```python
from build123d import *

# Parameters (mm, degrees)
CROQUIS1_R                                           = 32.7
CROQUIS1_R_2                                         = 5
SALIENTE_EXTRUIR1_DEPTH                              = 4.25
REFRENTADO_PARA_TORNILLO_CON_CABEZA_TRON_D           = 3.4
REFRENTADO_PARA_TORNILLO_CON_CABEZA_TRON_CBORE_D     = 7
REFRENTADO_PARA_TORNILLO_CON_CABEZA_TRON_CBORE_DEPTH = 2.4
CROQUIS5_R                                           = 32.7
CROQUIS5_R_2                                         = 21.5
SALIENTE_EXTRUIR2_DEPTH                              = 55
TALADRO_DE_MARGEN_PARA_M31_D                         = 3.4
TALADRO_DE_MARGEN_PARA_M31_DEPTH                     = 15
TALADRO_DE_MARGEN_PARA_M31_TIP                       = 1.021463052
TALADRO_DE_MARGEN_PARA_M32_D                         = 3.4
TALADRO_DE_MARGEN_PARA_M32_DEPTH                     = 16.5
TALADRO_DE_MARGEN_PARA_M32_TIP                       = 1.021463052
CROQUIS16_R                                          = 32.7
SALIENTE_EXTRUIR3_DEPTH                              = 7.5
SALIENTE_EXTRUIR4_START                              = -10
CROQUIS17_R                                          = 42.5
CROQUIS17_R_2                                        = 32.7
SALIENTE_EXTRUIR4_DEPTH                              = 10
REFRENTADO_PARA_TORNILLO_CON_CABEZA_2_D              = 3.4
REFRENTADO_PARA_TORNILLO_CON_CABEZA_2_CBORE_D        = 7
REFRENTADO_PARA_TORNILLO_CON_CABEZA_2_CBORE_DEPTH    = 2.4


with BuildPart() as part:
    # Croquis1 → Saliente-Extruir1 (new, symmetric)
    with BuildSketch(Plane(origin=(0, 0, 0), x_dir=(0, 0, -1), z_dir=(1, 0, 0))):
        Circle(CROQUIS1_R)
        Circle(CROQUIS1_R_2, mode=Mode.SUBTRACT)
    extrude(amount=SALIENTE_EXTRUIR1_DEPTH, both=True)

    # Refrentado para tornillo con cabeza tron (through all)
    with Locations(Plane(origin=(4.25, 0, 0), x_dir=(0, 0, -1), z_dir=(1, 0, 0))):
        with Locations((8.838834765, 8.838834765), (-8.838834765, -8.838834765), (-8.838834765, 8.838834765), (8.838834765, -8.838834765)):
            CounterBoreHole(REFRENTADO_PARA_TORNILLO_CON_CABEZA_TRON_D / 2, REFRENTADO_PARA_TORNILLO_CON_CABEZA_TRON_CBORE_D / 2, REFRENTADO_PARA_TORNILLO_CON_CABEZA_TRON_CBORE_DEPTH)

    # Croquis5 → Saliente-Extruir2 (add)
    with BuildSketch(Plane.ZY.offset(4.25)):
        Circle(CROQUIS5_R)
        Circle(CROQUIS5_R_2, mode=Mode.SUBTRACT)
    extrude(amount=SALIENTE_EXTRUIR2_DEPTH)

    # Taladro de margen para M31
    with Locations(Plane.ZY.offset(59.25)):
        with Locations((17.075, 17.075), (-17.075, -17.075), (-17.075, 17.075), (17.075, -17.075)):
            Hole(TALADRO_DE_MARGEN_PARA_M31_D / 2, depth=TALADRO_DE_MARGEN_PARA_M31_DEPTH)
            with Locations((0, 0, -(TALADRO_DE_MARGEN_PARA_M31_DEPTH + TALADRO_DE_MARGEN_PARA_M31_TIP / 2))):  # 118° drill point
                Cone(0, TALADRO_DE_MARGEN_PARA_M31_D / 2, TALADRO_DE_MARGEN_PARA_M31_TIP, mode=Mode.SUBTRACT)

    # Taladro de margen para M32
    with Locations(Plane(origin=(4.25, 0, 0), x_dir=(0, 0, -1), z_dir=(1, 0, 0))):
        with Locations((15.5, 15.5), (-15.5, -15.5), (-15.5, 15.5), (15.5, -15.5)):
            Hole(TALADRO_DE_MARGEN_PARA_M32_D / 2, depth=TALADRO_DE_MARGEN_PARA_M32_DEPTH)
            with Locations((0, 0, -(TALADRO_DE_MARGEN_PARA_M32_DEPTH + TALADRO_DE_MARGEN_PARA_M32_TIP / 2))):  # 118° drill point
                Cone(0, TALADRO_DE_MARGEN_PARA_M32_D / 2, TALADRO_DE_MARGEN_PARA_M32_TIP, mode=Mode.SUBTRACT)

    # Croquis16 → Saliente-Extruir3 (add)
    with BuildSketch(Plane.ZY.offset(59.25)):
        Circle(CROQUIS16_R)
        with BuildLine():
            Line((-16.5, 21.5), (16.5, 21.5))
            ThreePointArc((16.5, 21.5), (20.035533906, 20.035533906), (21.5, 16.5))
            Line((21.5, 16.5), (21.5, -16.5))
            ThreePointArc((21.5, -16.5), (20.035533906, -20.035533906), (16.5, -21.5))
            Line((16.5, -21.5), (-16.5, -21.5))
            ThreePointArc((-16.5, -21.5), (-20.035533906, -20.035533906), (-21.5, -16.5))
            Line((-21.5, -16.5), (-21.5, 16.5))
            ThreePointArc((-21.5, 16.5), (-20.035533906, 20.035533906), (-16.5, 21.5))
        make_face(mode=Mode.SUBTRACT)
    extrude(amount=SALIENTE_EXTRUIR3_DEPTH)

    # Croquis17 → Saliente-Extruir4 (add)
    with BuildSketch(Plane.ZY.offset(66.75).offset(SALIENTE_EXTRUIR4_START)):
        Circle(CROQUIS17_R)
        Circle(CROQUIS17_R_2, mode=Mode.SUBTRACT)
    extrude(amount=SALIENTE_EXTRUIR4_DEPTH)

    # Refrentado para tornillo con cabeza  2 (through all)
    with Locations(Plane(origin=(-56.75, 0, 0), x_dir=(0, 0, -1), z_dir=(1, 0, 0))):
        with Locations((0, 37.6), (26.587214973, 26.587214973), (37.6, 0), (26.587214973, -26.587214973), (0, -37.6), (-26.587214973, -26.587214973), (-37.6, 0), (-26.587214973, 26.587214973)):
            CounterBoreHole(REFRENTADO_PARA_TORNILLO_CON_CABEZA_2_D / 2, REFRENTADO_PARA_TORNILLO_CON_CABEZA_2_CBORE_D / 2, REFRENTADO_PARA_TORNILLO_CON_CABEZA_2_CBORE_DEPTH)


solid = part.part
```
Design review of the part built by this model. Coordinates are the model's own, in mm. A direction names the side the tool comes from. Give positions to 0.01 mm unless a question says otherwise; leave off trailing zeros. Loops run counter-clockwise (first coordinate to the right, second up) from the corner with the lowest first, then second, coordinate; pieces in that order, holes last. Notation, with made-up numbers: (-10, 23.5) -> (11, 23.5) arc R19 ccw to (11, 28.5) -> close; hole circle Ø11 at (-5, 30). An arc over 180 degrees is marked (long way). Write each question's results on one line, items separated by ' | '.
Q1. Take a section at A-A, the plane z = 27. Write out the cut boundary in (x, y), plus the area to 3 significant figures.
Reply:
outline: (-66.75, -32.82) -> (-56.75, -32.82) -> (-56.75, -30.06) -> (-59.15, -30.06) -> (-59.15, -28.24) -> (-66.75, -28.24) -> close; (-66.75, -24.94) -> (-59.15, -24.94) -> (-59.15, -23.11) -> (-56.75, -23.11) -> (-56.75, -18.45) -> (4.25, -18.45) -> (4.25, 18.45) -> (-56.75, 18.45) -> (-56.75, 23.11) -> (-59.15, 23.11) -> (-59.15, 24.94) -> (-66.75, 24.94) -> close; (-66.75, 28.24) -> (-59.15, 28.24) -> (-59.15, 30.06) -> (-56.75, 30.06) -> (-56.75, 32.82) -> (-66.75, 32.82) -> close | area: 2,820 mm²
Q2. Wall thickness on L1, parallel to Y at x = -64, z = 0; L2, parallel to Y at x = -60.5, z = 1; L3, parallel to Z at x = -3, y = 15: over which ranges is each line inside the solid? List them lowest first.
Reply:
L1: y = -42.5 to -39.3, -35.9 to -21.5, 21.5 to 35.9, 39.3 to 42.5 | L2: y = -42.49 to -38.97, -36.23 to -21.5, 21.5 to 36.23, 38.97 to 42.49 | L3: z = -29.06 to -17.12, -13.88 to 13.88, 17.12 to 29.06
Q3. Take a section at D-D, the plane x = -26. Write out the cut boundary in (y, z), plus the area to 3 significant figures.
Reply:
outline: circle Ø65.4 at (0, 0); hole circle Ø43 at (0, 0) | area: 1,910 mm²
Q4. For pin 1 Ø6 at (x, z) = (-14.5, 27) entering from -Y; pin 2 Ø2 at (y, z) = (-15.5, 15.5) entering from -X; pin 3 Ø11 at (y, z) = (-26.59, 26.59) entering from -X; pin 4 Ø3.5 at (y, z) = (-9.5, 8.5) entering from +X, all flat-tipped, find the tip position at first contact; note any pin that passes through.
Reply:
pin 1: stops at y = -22.21 | pin 2: stops at x = -59.25 | pin 3: stops at x = -66.75 | pin 4: stops at x = 1.85
Q5. Machinability: for faces 1 (the face through (-0.06, -4.88, 1.08)), 2 (the face through (-59.15, -37, -2)), 3 (the face through (-59.25, 16, 15)), which of the approach directions +Z, -Z, +X, -X, +Y, -Y give a long, thin tool a straight path to every point of the face, cutting with its end or side? Answer none if there is none.
Reply:
face 1: +X, -X | face 2: +X | face 3: -X
Q6. The part is to be moulded in two halves that separate along Y. For faces 4 (the face through (-12.98, 15.91, -15.76)), 5 (the face through (-66.75, 1, 28)), 6 (the face through (-4.12, -16.15, 17.07)), 7 (the face through (-61.68, -25.861, -33.727)), say which applies: +Y half, -Y half, draft (parallel to the pull), parting line (faces both ways), or undercut.
Reply:
face 4: undercut | face 5: draft | face 6: undercut | face 7: parting line
Q7. Take a section at B-B, the plane y = -37.6. Write out the cut boundary in (x, z), plus the area to 3 significant figures.
Reply:
outline: (-66.75, -19.81) -> (-56.75, -19.81) -> (-56.75, -3.5) -> (-59.15, -3.5) -> (-59.15, -1.7) -> (-66.75, -1.7) -> close; (-66.75, 1.7) -> (-59.15, 1.7) -> (-59.15, 3.5) -> (-56.75, 3.5) -> (-56.75, 19.81) -> (-66.75, 19.81) -> close | area: 354 mm²
